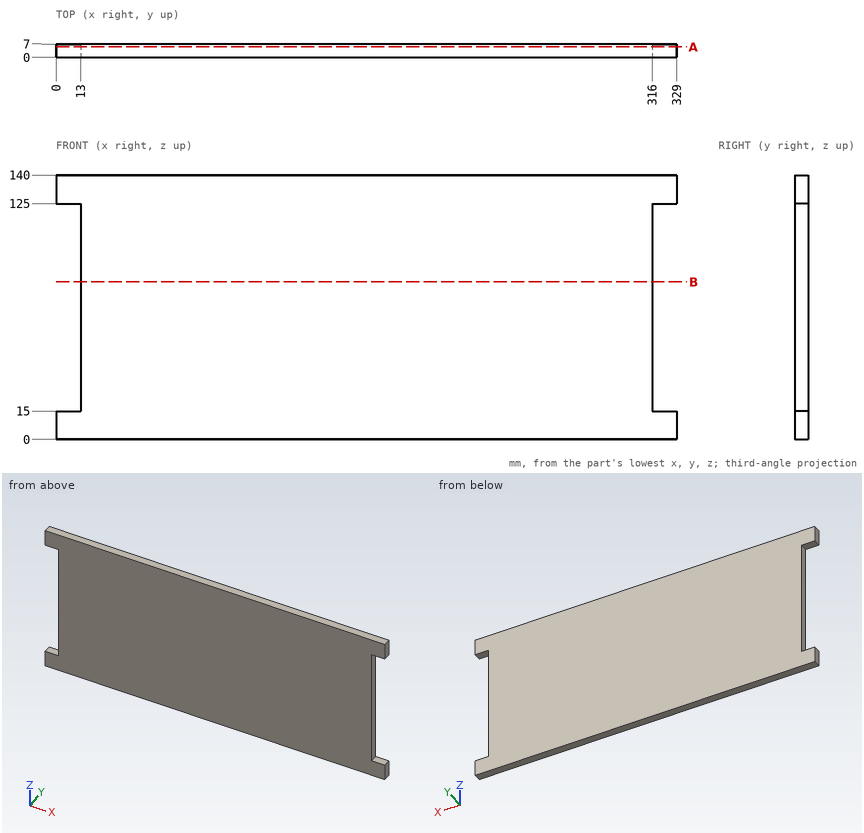
Part print with two shaded views. Sizes in mm from the minimum x, y, z corner. Round coordinates to 2 decimals unless told otherwise and drop trailing zeros. Loops run counter-clockwise (first coordinate to the right, second up) from the corner with the lowest first, then second, coordinate; pieces in that order, holes last.
1. Drill centre line: line 1 along X through (y, z) = (1.25, 107). Where is it in solid material? Low to high.
Solutions:
line 1: x = 13 to 316
2. Slice it at B-B (z = 83.5). Give the cut face in (x, y).
Solutions:
outline: (13, 0) - (316, 0) - (316, 7) - (13, 7) - close
3. Slice it at A-A (y = 5.5). Give the cut face in (x, z), and give its area (3 significant figures).
Solutions:
outline: (0, 0) - (329, 0) - (329, 15) - (316, 15) - (316, 125) - (329, 125) - (329, 140) - (0, 140) - (0, 125) - (13, 125) - (13, 15) - (0, 15) - close
area: 43,200 mm2
4. Flat gauge pins, fed straight in: pin 1 (3.5 mm diameter, centred on x = 4, y = 3, fed in from -Z); pin 2 (1 mm diameter, centred on y = 4.5, z = 23, fed in from +X); pin 3 (2 mm diameter, centred on y = 2.5, z = 60.5, fed in from -X). Where does each tip first touch, or does it go through?
Solutions:
pin 1: stops at z = 0
pin 2: stops at x = 316
pin 3: stops at x = 13
